Can you work these out from the model? Positions are in its coordinate system, mm. A direction names the side the tool comes from. Give positions to 0.01 mm unless a question says otherwise; leave off trailing zeros. Loops run counter-clockwise (first coordinate to the right, second up) from the corner with the lowest first, then second, coordinate; pieces in that order, holes last. Notation, with made-up numbers: M 40.25,13.5 L 85.25,13.5 A27 ccw 85.25,31.5 Z; hole C 34,55 d3. An arc over 180 degrees is marked long. One line per item, written item: value. Start each with the question number.
from build123d import *

# Parameters (mm, degrees)
SALIENTE_EXTRUIR1_DEPTH = 5
SALIENTE_EXTRUIR2_DEPTH = 5


with BuildPart() as part:
    # Croquis1 → Saliente-Extruir1 (new body)
    with BuildSketch(Plane.XY):
        with BuildLine():
            ThreePointArc((-51.659530699, 2.243564356), (0, -40.9), (51.659530699, 2.243564356))
            ThreePointArc((51.659530699, 2.243564356), (51.226617189, 3.88201574), (49.691548577, 4.6))
            Line((49.691548577, 4.6), (-49.691548577, 4.6))
            ThreePointArc((-49.691548577, 4.6), (-51.226617189, 3.88201574), (-51.659530699, 2.243564356))
        make_face()
        with BuildLine():
            ThreePointArc((-3.5, -31.457984161), (-25.58189602, -23.211012568), (-40.04747183, -4.6))
            Line((-40.04747183, -4.6), (-5.5, -4.6))
            Line((-5.5, -4.6), (-5.5, -9.6))
            ThreePointArc((-5.5, -9.6), (-4.977225575, -12.049489743), (-3.5, -14.072135955))
            Line((-3.5, -14.072135955), (-3.5, -31.457984161))
        make_face(mode=Mode.SUBTRACT)
        with BuildLine():
            ThreePointArc((40.04747183, -4.6), (25.984811469, -22.911296309), (4.5, -31.364985744))
            Line((4.5, -31.364985744), (4.5, -14.072135955))
            ThreePointArc((4.5, -14.072135955), (5.977225575, -12.049489743), (6.5, -9.6))
            Line((6.5, -9.6), (6.5, -4.6))
            Line((6.5, -4.6), (40.04747183, -4.6))
        make_face(mode=Mode.SUBTRACT)
        with BuildLine():
            Line((-3.5, -1.6), (-37, -1.6))
            Line((-37, -1.6), (-37, 1.6))
            Line((-37, 1.6), (37, 1.6))
            Line((37, 1.6), (37, -1.6))
            Line((37, -1.6), (4.5, -1.6))
            Line((4.5, -1.6), (4.5, -9.6))
            ThreePointArc((4.5, -9.6), (0.5, -13.6), (-3.5, -9.6))
            Line((-3.5, -9.6), (-3.5, -1.6))
        make_face(mode=Mode.SUBTRACT)
    extrude(amount=SALIENTE_EXTRUIR1_DEPTH)

    # Croquis3 → Saliente-Extruir2 (add)
    with BuildSketch(Plane.XY):
        with BuildLine():
            Line((40.04747183, -4.6), (6.5, -4.6))
            Line((6.5, -4.6), (6.5, -9.6))
            ThreePointArc((6.5, -9.6), (5.977225575, -12.049489743), (4.5, -14.072135955))
            Line((4.5, -14.072135955), (4.5, -31.364985744))
            ThreePointArc((4.5, -31.364985744), (10.160094866, -30.388242072), (15.640583324, -28.66924575))
            ThreePointArc((15.640583324, -28.66924575), (13.021749092, -7.49311258), (31.780404624, -17.661679411))
            ThreePointArc((31.780404624, -17.661679411), (36.502915311, -11.503618196), (40.04747183, -4.6))
        make_face()
        with BuildLine():
            Line((-3.5, -31.457984161), (-3.5, -14.072135955))
            ThreePointArc((-3.5, -14.072135955), (-4.977225575, -12.049489743), (-5.5, -9.6))
            Line((-5.5, -9.6), (-5.5, -4.6))
            Line((-5.5, -4.6), (-40.04747183, -4.6))
            ThreePointArc((-40.04747183, -4.6), (-36.502915311, -11.503618196), (-31.780404624, -17.661679411))
            ThreePointArc((-31.780404624, -17.661679411), (-13.021749092, -7.49311258), (-15.640583324, -28.66924575))
            ThreePointArc((-15.640583324, -28.66924575), (-9.671336411, -30.50350641), (-3.5, -31.457984161))
        make_face()
    extrude(amount=SALIENTE_EXTRUIR2_DEPTH)


solid = part.part
Q1. I need wall thicknesses on line 1 along X through (y, z) = (-18.5, 0.65); line 2 along X through (y, z) = (-13, 1.4); line 3 along X through (y, z) = (-25.5, 2.25). Which ranges of each line are inside material? Lowest first, please.
Q2. If we section it at D-D, the plane x = -29: Write out the boundary of the cut face in (y, z).
Q3. For P1, Ø1.5, axis at y = -7, z = 3.5, coming from the +X side; P2, Ø2.5, axis at y = 0, z = 3, coming from the -X side; P3, Ø2.5, axis at y = -0.5, z = 1.5, coming from the +X side, each with a flat end and sliding along its axis, tell me the tip position at first contact or that it passes through.
Q4. If we section it at A-A, the plane y = -21: Write out the boundary of the cut face in (x, z).
Q5. If we mould it in two halves opening along Y, with no side actions, what happens to faces 1 (the face through (-37, 0, 2)), 2 (the face through (-1.02, -40.89, 2.46)), 3 (the face through (-1, -18, 0))? For each: released by +Y, released by -Y, zero draft, split by the parting line, or undercut.
Q6. Which directions (+Z, -Z, +X, -X, +Y, -Y) give clear straight access to the entire face, cutting with the end or side of a thin tool? Please do faces 4 (the face through (1, 4.6, 2)), 5 (the face through (-24.227, -24.167, 2.465)).
Q7. If we section it at C-C, the plane z = 3.6: Write out the boundary of the cut face in (x, y).
Q8. If we section it at B-B, the plane x = 0.5: Write out the boundary of the cut face in (y, z), plus the area to 3 significant figures.
Response:
1. line 1: -43.01 to -30.99, -7.83 to 7.83, 30.99 to 43.01
1. line 2: -46.38 to -30.94, -8.62 to -1.61, 2.61 to 8.62, 30.94 to 46.38
1. line 3: -37.15 to -22.13, -10.92 to 10.92, 22.13 to 37.15
2. outline: M -32.16,0 L -20.42,0 L -20.42,5 L -32.16,5 Z; M -9.72,0 L -1.6,0 L -1.6,5 L -9.72,5 Z; M 1.6,0 L 4.6,0 L 4.6,5 L 1.6,5 Z
3. P1: x = 49.37
3. P2: x = -51.47
3. P3: x = 51.37
4. outline: M -41.15,0 L -28.35,0 L -28.35,5 L -41.15,5 Z; M -8.33,0 L 8.33,0 L 8.33,5 L -8.33,5 Z; M 28.35,0 L 41.15,0 L 41.15,5 L 28.35,5 Z
5. face 1: undercut
5. face 2: released by -Y
5. face 3: zero draft
6. face 4: +Z, -Z, +X, -X, +Y
6. face 5: +Z, -Z
7. outline: M -51.66,2.24 A52.5 ccw 51.66,2.24 A2 ccw 49.69,4.6 L -49.69,4.6 A2 ccw Z; hole M -37,-1.6 L -3.5,-1.6 L -3.5,-9.6 A4 ccw 4.5,-9.6 L 4.5,-1.6 L 37,-1.6 L 37,1.6 L -37,1.6 Z; hole M -31.78,-17.66 A43.2 ccw -15.64,-28.67 A12 ccw long Z; hole M 15.64,-28.67 A43.2 ccw 31.78,-17.66 A12 ccw long Z
8. outline: M -40.9,0 L -13.6,0 L -13.6,5 L -40.9,5 Z; M 1.6,0 L 4.6,0 L 4.6,5 L 1.6,5 Z
8. area: 151 mm^2
